Source: CAD feature listing. Evaluate the final solid. Frame: model axes, mm. Face numbers are marked on the shaded views. Give positions to 0.01 mm unless a question says otherwise; leave off trailing zeros. Put each result on its own line as item: value.
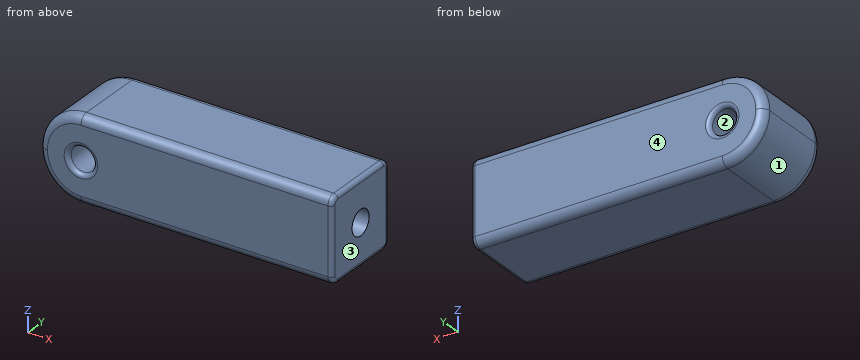
```python
from build123d import *

# Parameters (mm, degrees)
CROQUIS1_W              = 175
CROQUIS1_H              = 50
SALIENTE_EXTRUIR1_DEPTH = 50
REDONDEO1_R             = 25
CROQUIS2_R              = 7.5
CORTAR_EXTRUIR1_DEPTH   = 15
CROQUIS3_R              = 7.5
CORTAR_EXTRUIR2_DEPTH   = 189.745860882
REDONDEO2_R             = 5
REDONDEO3_R             = 2.5
REDONDEO4_R             = 2.5


with BuildPart() as part:
    # Croquis1 → Saliente-Extruir1 (new body)
    with BuildSketch(Plane.XY):
        with Locations((87.5, 25)):
            Rectangle(CROQUIS1_W, CROQUIS1_H)
    extrude(amount=SALIENTE_EXTRUIR1_DEPTH)

    # Redondeo1
    redondeo1_edges = [part.edges().sort_by_distance(p)[0] for p in [
        (0, 25, 0),
        (0, 25, 50),
    ]]
    fillet(redondeo1_edges, radius=REDONDEO1_R - 0.0001)  # a hair under: the kernel refuses the full size

    # Croquis2 → Cortar-Extruir1 (cut)
    with BuildSketch(Plane(origin=(175, 0, 0), x_dir=(0, 0, -1), z_dir=(1, 0, 0))):
        with Locations((-25, 25)):
            Circle(CROQUIS2_R)
    extrude(amount=-CORTAR_EXTRUIR1_DEPTH, mode=Mode.SUBTRACT)

    # Croquis3 → Cortar-Extruir2 (cut, through all)
    with BuildSketch(Plane(origin=(0, 50, 0), x_dir=(1, 0, 0), z_dir=(0, 1, 0))):
        with Locations(Location((25, -25, 0), (0, 0, 270))):
            Circle(CROQUIS3_R)
    extrude(amount=-CORTAR_EXTRUIR2_DEPTH, mode=Mode.SUBTRACT)

    # Redondeo2
    redondeo2_edges = [part.edges().sort_by_distance(p)[0] for p in [
        (99.99995, 50, 50),
        (99.99995, 0, 0),
        (99.99995, 0, 50),
        (7.322301181, 0, 42.677698819),
        (7.322301181, 0, 7.322301181),
        (7.322301181, 50, 42.677698819),
        (7.322301181, 50, 7.322301181),
        (99.99995, 50, 0),
    ]]
    fillet(redondeo2_edges, radius=REDONDEO2_R)

    # Redondeo3
    redondeo3_edges = [part.edges().sort_by_distance(p)[0] for p in [
        (25, 0, 17.5),
        (25, 50, 17.5),
    ]]
    fillet(redondeo3_edges, radius=REDONDEO3_R)

    # Redondeo4
    redondeo4_edges = [part.edges().sort_by_distance(p)[0] for p in [
        (175, 0, 25),
        (175, 50, 25),
        (175, 25, 0),
        (175, 25, 50),
        (175, 48.535533906, 48.535533906),
        (175, 48.535533906, 1.464466094),
        (175, 1.464466094, 48.535533906),
        (175, 1.464466094, 1.464466094),
    ]]
    fillet(redondeo4_edges, radius=REDONDEO4_R)


solid = part.part
```
1) Pin query (flat end, axial travel): P1, Ø4.5, axis at y = 25, z = 24, coming from the +X side. Return the tip coordinate at first contact, or that it passes through.
Check result:
P1: x = 160
2) Mould query, pull axis X, two halves, no side actions, for the marked faces 1, 2, 3 and 4. Classes: pulls with the +X half, pulls with the -X half, needs draft (parallel to the pull), parting line crosses it, or undercut.
Check result:
face 1: pulls with the -X half
face 2: undercut
face 3: pulls with the +X half
face 4: needs draft
3) Material intervals for line 1 along X through (y, z) = (15, 25); line 2 along Y through (x, z) = (168, 25); line 3 along X through (y, z) = (28, 25), sorted ascending. Write a range as [from, to].
Check result:
line 1: [0, 17.5], [32.5, 175]
line 2: [0, 17.5], [32.5, 50]
line 3: [0, 17.5], [32.5, 160]
